Verification items for the finished model (mm, model axes). Face numbers are marked on the shaded views. A direction names the side the tool comes from. Give positions to 0.01 mm unless a question says otherwise; leave off trailing zeros. Loops run counter-clockwise (first coordinate to the right, second up) from the corner with the lowest first, then second, coordinate; pieces in that order, holes last. Notation, with made-up numbers: (36, -29) - (78, -29) arc R21 cw to (78, -25) - close; hole circle Ø10 at (56, 58.25). An arc over 180 degrees is marked (long way). Put each result on its own line as item: value. Start each with the question number.
```python
from build123d import *

# Parameters (mm, degrees)
F1_DEPTH       = 8
F3_D           = 4
F3_CSINK_D     = 5
F3_CSINK_ANGLE = 90
F4_R           = 1


with BuildPart() as f1:
    # F0 (on Front) → F1 (new body, symmetric)
    with BuildSketch(Plane.XZ):
        with BuildLine():
            Line((-24.75, -5.63766), (24.75, -5.63766))
            Line((24.75, -5.63766), (24.75, 2.36234))
            Line((24.75, 2.36234), (12.75, 2.36234))
            Line((12.75, 2.36234), (12.75, 38.36234))
            Line((12.75, 38.36234), (0.75, 38.36234))
            Line((0.75, 38.36234), (0.75, 31.327106))
            ThreePointArc((0.75, 31.327106), (0, 15.36234), (-0.75, 31.327106))
            Line((-0.75, 31.327106), (-0.75, 38.36234))
            Line((-0.75, 38.36234), (-12.75, 38.36234))
            Line((-12.75, 38.36234), (-12.75, 2.36234))
            Line((-12.75, 2.36234), (-24.75, 2.36234))
            Line((-24.75, 2.36234), (-24.75, -5.63766))
        make_face()
    extrude(amount=F1_DEPTH, both=True)

    # F3 (through all)
    with Locations(Plane.XY.offset(2.36234)):
        with Locations((18.75, 0), (-18.75, 0)):
            CounterSinkHole(F3_D / 2, F3_CSINK_D / 2, counter_sink_angle=F3_CSINK_ANGLE)

    # F4
    f4_edges = [f1.edges().sort_by_distance(p)[0] for p in [
        (-12.75, -8, 20.36234),
        (-18.75, -8, 2.36234),
        (-24.75, -8, -1.63766),
        (-6.75, -8, 38.36234),
        (6.75, -8, 38.36234),
        (12.75, -8, 20.36234),
        (18.75, -8, 2.36234),
        (24.75, -8, -1.63766),
        (0, -8, 15.36234),
        (24.75, 8, -1.63766),
        (18.75, 8, 2.36234),
        (12.75, 8, 20.36234),
        (6.75, 8, 38.36234),
        (-6.75, 8, 38.36234),
        (-12.75, 8, 20.36234),
        (-18.75, 8, 2.36234),
        (-24.75, 8, -1.63766),
        (0, 8, 15.36234),
        (12.75, 0, 2.36234),
        (24.75, 0, 2.36234),
        (12.75, 0, 38.36234),
        (-24.75, 0, 2.36234),
        (-12.75, 0, 2.36234),
        (-12.75, 0, 38.36234),
    ]]
    fillet(f4_edges, radius=F4_R)


solid = f1.part
```
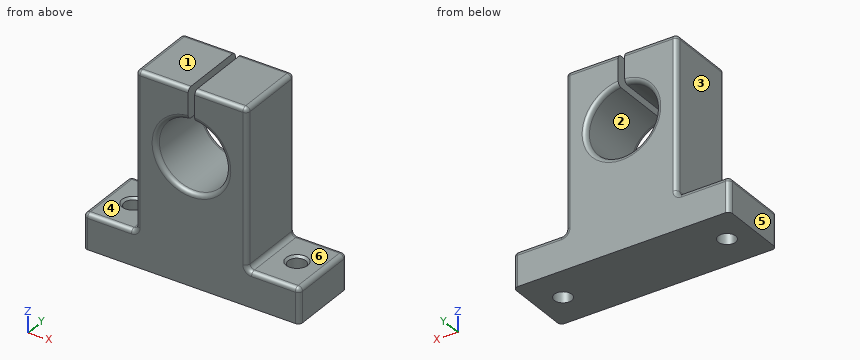
1) Section check B-B, the plane x = 18.75. Enter the section's corners in (y, z), plus the area to 3 significant figures.
2) Section check D-D, the plane y = -5.25. Enter the section's corners in (x, z).
3) Draft check along X on the marked faces 1, 2 and 3. Enter one of: pulls with the +X half, pulls with the -X half, needs draft (parallel to the pull), parting line crosses it, or undercut.
4) Section check C-C, the plane x = 0. Enter the section's corners in (y, z).
5) Section check A-A, the plane y = 0. State how many separate pieces and enclosed holes the cut face has, plus the area to 3 significant figures.
6) Scan lines: line 1 along X through (y, z) = (0, -3.5); line 2 along Y through (x, z) = (18.75, -0.5); line 3 along Z through (x, y) = (4.5, -4.75). Record each from-to range of solid material in increasing order. Write a range as from..to.
7) Depth check by flat-ended pin: P1, Ø3, axis at x = 21, y = -1, coming from the +Z side; P2, Ø2, axis at y = 0, z = 35, coming from the +X side; P3, Ø3.5, axis at y = 3.5, z = 34.5, coming from the -X side; P4, Ø3, axis at x = -18.75, y = 0, coming from the +Z side. Enter the tip coordinate at first touch or a pass-through.
8) Set-up check for the marked faces 4, 5 and 6: record each of +Z, -Z, +X, -X, +Y, -Y from which the full face is reachable in a straight line by a thin tool's end or side.
Results are:
1. outline: (-8, -5.64) - (-2, -5.64) - (-2, 1.86) - (-2.5, 2.36) - (-7, 2.36) arc R1 ccw to (-8, 1.36) - close; (2, -5.64) - (8, -5.64) - (8, 1.36) arc R1 ccw to (7, 2.36) - (2.5, 2.36) - (2, 1.86) - close
1. area: 95.3 mm2
2. outline: (-24.75, -5.64) - (24.75, -5.64) - (24.75, 1.36) arc R1 ccw to (23.75, 2.36) - (13.75, 2.36) arc R1 cw to (12.75, 3.36) - (12.75, 37.36) arc R1 ccw to (11.75, 38.36) - (0.75, 38.36) - (0.75, 31.33) arc R8 cw (long way) to (-0.75, 31.33) - (-0.75, 38.36) - (-11.75, 38.36) arc R1 ccw to (-12.75, 37.36) - (-12.75, 3.36) arc R1 cw to (-13.75, 2.36) - (-23.75, 2.36) arc R1 ccw to (-24.75, 1.36) - close
3. face 1: needs draft
3. face 2: undercut
3. face 3: pulls with the -X half
4. outline: (-8, -5.64) - (8, -5.64) - (8, 14.36) arc R1 ccw to (7, 15.36) - (-7, 15.36) arc R1 ccw to (-8, 14.36) - close
5. separate pieces: 3
5. enclosed holes: 0
5. area: 1,040 mm2
6. line 1: x = -24.75..-20.75, -16.75..16.75, 20.75..24.75
6. line 2: y = -8..-2, 2..8
6. line 3: z = -5.64..16.75, 29.98..38.36
7. P1: stops at z = 2.36
7. P2: stops at x = 12.75
7. P3: stops at x = -12.75
7. P4: passes through
8. face 4: +Z, -X, +Y, -Y
8. face 5: +Z, -Z, -X, +Y, -Y
8. face 6: +Z, +X, +Y, -Y
